Build history of the part. All positions in model axes, mm. Face numbers are marked on the shaded views. A direction names the side the tool comes from. Coordinates: 2 decimals unless noted, no trailing zeros. Order: outer loops, then holes, each group sorted by start corner. A loop starts at its lowest first (then second) coordinate and runs counter-clockwise, first axis right, second up. Notation, with made-up numbers: (81.25, 21.5) - (95.25, 21.5) arc R21 cw to (95.25, 47.5) - close; hole circle Ø5 at (89, 43.5). An arc over 180 degrees is marked (long way). Return JSON: item names as keys, results as strings.
from build123d import *

# Parameters (mm, degrees)
EXTRUDE_6_DEPTH        = 34
EXTRUDE_7_REACH        = 108.193
EXTRUDE_7_END_RADIUS   = 26
SKETCH_15_R            = 12.5
EXTRUDE_8_REACH        = 150.176
EXTRUDE_8_END_RADIUS   = 26
SKETCH_16_W            = 68
SKETCH_16_H            = 12
EXTRUDE_9_DEPTH        = 8
FILLET_2_R             = 10
EXTRUDE_10_DEPTH       = 19
CUT_EXTRUDE_7_DEPTH    = 8
SKETCH_20_R            = 17.5
CUT_EXTRUDE_8_DEPTH    = 68
CUT_EXTRUDE_9_REACH    = 136.108
SKETCH_21_R            = 17.5
CUT_EXTRUDE_10_DEPTH   = 5
CUT_EXTRUDE_11_DEPTH   = 9
CUT_EXTRUDE_12_DEPTH   = 4
FILLET_3_R             = 3
HOLE_WIZARD_M8_1_D     = 6.8
HOLE_WIZARD_M8_1_DEPTH = 15.75
HOLE_WIZARD_M8_1_TIP   = 2.042926105


with BuildPart() as part:
    # 草图1 → 凸台-拉伸6 (new, symmetric)
    with BuildSketch(Plane(origin=(0, 0, 0), x_dir=(0, 0, -1), z_dir=(1, 0, 0))):
        with BuildLine():
            Line((-18, -22), (-13.856406461, -22))
            ThreePointArc((-13.856406461, -22), (9.116890708, 24.349174602), (-4, -25.690465157))
            Line((-4, -25.690465157), (-4, -80))
            Line((-4, -80), (-18, -80))
            Line((-18, -80), (-18, -22))
        make_face()
    extrude(amount=EXTRUDE_6_DEPTH, both=True)

    # 凸台-拉伸7: up to this cylinder (the profile starts outside it)
    extrude_7_end = Plane(origin=(0, 0, 0), z_dir=(-1, 0, 0)) * Cylinder(EXTRUDE_7_END_RADIUS, 269.386, mode=Mode.PRIVATE)
    # 草图15 → 凸台-拉伸7 (add, up to the surface)
    with BuildSketch(Plane.XY.offset(35), mode=Mode.PRIVATE) as extrude_7_sk1:
        with Locations((0, 13.5)):
            Circle(SKETCH_15_R)
    extrude_7_tool1 = extrude(extrude_7_sk1.sketch, amount=-EXTRUDE_7_REACH, mode=Mode.PRIVATE) - extrude_7_end
    add(extrude_7_tool1.solids().sort_by_distance((0, 13.5, 35))[0])

    # 凸台-拉伸8: up to this cylinder (the profile starts outside it)
    extrude_8_end = Plane(origin=(0, 0, 0), z_dir=(-1, 0, 0)) * Cylinder(EXTRUDE_8_END_RADIUS, 353.352, mode=Mode.PRIVATE)
    # 草图16 → 凸台-拉伸8 (add, up to the surface)
    with BuildSketch(Plane.XY.offset(-85), mode=Mode.PRIVATE) as extrude_8_sk1:
        with Locations((0, 12)):
            Rectangle(SKETCH_16_W, SKETCH_16_H)
    extrude_8_tool1 = extrude(extrude_8_sk1.sketch, amount=EXTRUDE_8_REACH, mode=Mode.PRIVATE) - extrude_8_end
    add(extrude_8_tool1.solids().sort_by_distance((0, 12, -85))[0])

    # 草图17 → 凸台-拉伸9 (add)
    with BuildSketch(Plane(origin=(34, 0, 0), x_dir=(0, 0, -1), z_dir=(1, 0, 0))):
        with BuildLine():
            Line((-4, -34.770677301), (-4, -25.690465157))
            ThreePointArc((-4, -25.690465157), (19.091227119, -17.650072155), (25.298221281, 6))
            Line((25.298221281, 6), (34.481879299, 6))
            ThreePointArc((34.481879299, 6), (25.452863755, -24.023982324), (-4, -34.770677301))
        make_face()
    extrude_9 = extrude(amount=-EXTRUDE_9_DEPTH)

    # 镜向2: 凸台-拉伸9 across plane
    add(extrude_9.mirror(Plane(origin=(0, 0, 0), x_dir=(0, 0, 1), z_dir=(1, 0, 0))))

    # 圆角2
    fillet_2_edges = [part.edges().sort_by_distance(p)[0] for p in [
        (30, -34.770677301, 4),
        (-30, -34.770677301, 4),
    ]]
    fillet(fillet_2_edges, radius=FILLET_2_R)

    # 草图18 → 凸台-拉伸10 (add)
    with BuildSketch(Plane(origin=(0, 26, 0), x_dir=(1, 0, 0), z_dir=(0, 1, 0))):
        with BuildLine():
            Line((-18, 59), (-18, 18.761663039))
            ThreePointArc((-18, 18.761663039), (0, -26), (18, 18.761663039))
            Line((18, 18.761663039), (18, 59))
            ThreePointArc((18, 59), (0, 77), (-18, 59))
        make_face()
    extrude(amount=-EXTRUDE_10_DEPTH)

    # 草图19 → 切除-拉伸7 (cut)
    with BuildSketch(Plane(origin=(0, 26, 0), x_dir=(1, 0, 0), z_dir=(0, 1, 0))):
        with BuildLine():
            Line((-10, 59), (-10, 14.361406616))
            ThreePointArc((-10, 14.361406616), (0, -17.5), (10, 14.361406616))
            Line((10, 14.361406616), (10, 59))
            ThreePointArc((10, 59), (0, 69), (-10, 59))
        make_face()
    extrude(amount=-CUT_EXTRUDE_7_DEPTH, mode=Mode.SUBTRACT)

    # 草图20 → 切除-拉伸8 (cut)
    with BuildSketch(Plane(origin=(34, 0, 0), x_dir=(0, 0, -1), z_dir=(1, 0, 0))):
        Circle(SKETCH_20_R)
    extrude(amount=-CUT_EXTRUDE_8_DEPTH, mode=Mode.SUBTRACT)

    # 草图21 → 切除-拉伸9 (cut, up to next)
    with BuildSketch(Plane(origin=(0, 18, 0), x_dir=(1, 0, 0), z_dir=(0, 1, 0)), mode=Mode.PRIVATE) as cut_extrude_9_sk1:
        with Locations(Location((0, 0, 0), (0, 0, 270))):
            Circle(SKETCH_21_R)
    cut_extrude_9_tool1 = extrude(cut_extrude_9_sk1.sketch, amount=-CUT_EXTRUDE_9_REACH, mode=Mode.PRIVATE) & part.part
    add(cut_extrude_9_tool1.solids().sort_by_distance((0, 18, 0))[0], mode=Mode.SUBTRACT)

    # 草图22 → 切除-拉伸10 (cut)
    with BuildSketch(Plane.XY.offset(18)):
        with BuildLine():
            Line((-18, -45), (-18, -80))
            Line((-18, -80), (18, -80))
            Line((18, -80), (18, -45))
            ThreePointArc((18, -45), (0, -27), (-18, -45))
        make_face()
    extrude(amount=-CUT_EXTRUDE_10_DEPTH, mode=Mode.SUBTRACT)

    # 草图23 → 切除-拉伸11 (cut)
    with BuildSketch(Plane.XY.offset(13)):
        with BuildLine():
            Line((11, -80), (11, -45))
            ThreePointArc((11, -45), (0, -34), (-11, -45))
            Line((-11, -45), (-11, -80))
            Line((-11, -80), (11, -80))
        make_face()
    extrude(amount=-CUT_EXTRUDE_11_DEPTH, mode=Mode.SUBTRACT)

    # 草图24 → 切除-拉伸12 (cut)
    with BuildSketch(Plane(origin=(0, 26, 0), x_dir=(1, 0, 0), z_dir=(0, 1, 0))):
        with BuildLine():
            Line((0, 59), (-15.588457268, 68))
            ThreePointArc((-15.588457268, 68), (0, 77), (15.588457268, 68))
            Line((15.588457268, 68), (0, 59))
        make_face()
    extrude(amount=-CUT_EXTRUDE_12_DEPTH, mode=Mode.SUBTRACT)

    # 圆角3
    fillet_3_edges = [part.edges().sort_by_distance(p)[0] for p in [
        (34, 12, -85),
        (-34, 12, -85),
        (-34, -80, 11),
        (34, -80, 11),
    ]]
    fillet(fillet_3_edges, radius=FILLET_3_R)

    # M8 螺纹孔1
    with Locations(Plane(origin=(0, 13.5, 35), x_dir=(1, 0, 0), z_dir=(0, 0, 1))):
        with Locations((0, 0)):
            Hole(HOLE_WIZARD_M8_1_D / 2, depth=HOLE_WIZARD_M8_1_DEPTH)
            with Locations((0, 0, -(HOLE_WIZARD_M8_1_DEPTH + HOLE_WIZARD_M8_1_TIP / 2))):  # 118° drill point
                Cone(0, HOLE_WIZARD_M8_1_D / 2, HOLE_WIZARD_M8_1_TIP, mode=Mode.SUBTRACT)


solid = part.part
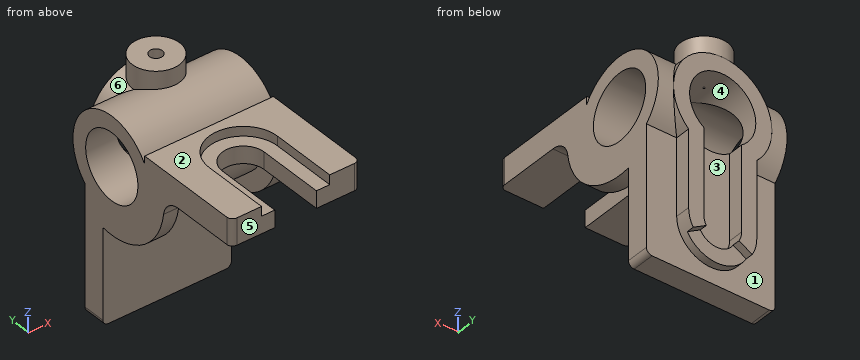
1. Tool access for the marked faces 1, 2 and 3: list every direction of +Z, -Z, +X, -X, +Y, -Y with a clear straight run to the whole face (end or side of a thin tool).
Check values:
{"face 1": "-Z, +Y", "face 2": "+Z, +X, -X, -Y", "face 3": "+Y"}
2. Cut at B-B on z = -43. Give the cut face in (x, y).
Check values:
{"outline": "(-34, 6) - (34, 6) - (34, 18) - (18, 18) - (18, 26) - (10, 26) - (10, 18) - (-10, 18) - (-10, 26) - (-18, 26) - (-18, 18) - (-34, 18) - close"}
3. Cut at D-D on y = -4. Give the cut face in (x, z), plus the area to 3 significant figures.
Check values:
{"outline": "(-34, -34.77) - (-26, -34.77) - (-26, -25.69) - (26, -25.69) - (26, -34.77) - (34, -34.77) - (34, -17.04) - (-34, -17.04) - close; (-34, 17.04) - (34, 17.04) - (34, 25.69) - (-34, 25.69) - close", "area": "1,320 mm²"}
4. Probe L1, parallel to X at y = -74, z = 14; L2, parallel to X at y = 13.5, z = 29.75; L3, parallel to Y at x = 10.5, z = -38. List the from-to ranges inside material, lowest first.
Check values:
{"L1": "-34 to -18, 18 to 34", "L2": "-12.5 to -3.4, 3.4 to 12.5", "L3": "6 to 26"}
5. Cut at A-A on y = -65.5. Give the cut face in (x, z).
Check values:
{"outline": "(-34, 4) - (-11, 4) - (-11, 13) - (-18, 13) - (-18, 18) - (-34, 18) - close; (11, 4) - (34, 4) - (34, 18) - (18, 18) - (18, 13) - (11, 13) - close"}
6. Drop flat-ended pins along their axis: pin 1 (1.2 mm diameter, centred on x = 6, z = 15, fed in from +Y); pin 2 (6.5 mm diameter, centred on y = 22.5, z = -39.5, fed in from +X); pin 3 (10 mm diameter, centred on x = 25.5, z = -48.5, fed in from -Y). Give the stop position or say it passes through.
Check values:
{"pin 1": "y = -7.93", "pin 2": "x = 18", "pin 3": "y = 6"}
7. Cut at C-C on x = -22.5. Give the cut face in (y, z).
Check values:
{"outline": "(-80, 4) - (-25.69, 4) arc R26 ccw to (6, -25.3) - (6, -85) - (18, -85) - (18, -18.76) arc R26 ccw to (22.5, -13.03) - (26, -13.03) - (26, 13.03) - (22.5, 13.03) arc R26 ccw to (-22, 13.86) - (-22, 18) - (-80, 18) - close; hole circle Ø35 at (0, 0)"}
8. Mould opens along X. For the marked faces 4, 5 and 6 say: pulls with the +X half, pulls with the -X half, needs draft (parallel to the pull), parting line crosses it, or undercut.
Check values:
{"face 4": "undercut", "face 5": "needs draft", "face 6": "pulls with the -X half"}
